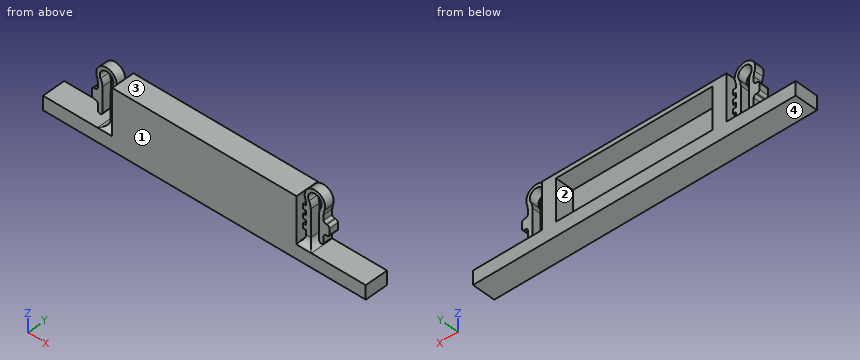
from build123d import *

# Parameters (mm, degrees)
BOSS_EXTRUDE1_DEPTH = 12.7
SKETCH6_W           = 86.36
SKETCH6_H           = 22.86
CUT_EXTRUDE3_DEPTH  = 10.16
SKETCH7_W           = 12.7
SKETCH7_H           = 25.4
CUT_EXTRUDE4_DEPTH  = 12.7
SKETCH14_W          = 88.9
SKETCH14_H          = 33.02
CUT_EXTRUDE5_DEPTH  = 19.558
BOSS_EXTRUDE2_START = -3.81
SKETCH15_W          = 2.54
SKETCH15_H          = 21.363451449
SKETCH15_W_2        = 3.175
SKETCH15_H_2        = 5.842
BOSS_EXTRUDE2_DEPTH = 5.08
FILLET1_R           = 7.62
FILLET2_R           = 1.27
FILLET3_R           = 3.81
BOSS_EXTRUDE3_START = -3.81
SKETCH16_W          = 1.778
SKETCH16_H          = 2.54
BOSS_EXTRUDE3_DEPTH = 5.08


# Some blends are built 0.0001 mm under size
with BuildPart() as part:
    # Sketch1 → Boss-Extrude1 (new body)
    with BuildSketch(Plane(origin=(0, 0, 0), x_dir=(1, 0, 0), z_dir=(0, 1, 0))):
        Polygon((88.9, 16.51), (-88.9, 16.51), (-88.9, 8.89), (-63.5, 8.89), (-63.5, -16.51), (63.5, -16.51), (63.5, 8.89), (88.9, 8.89), align=None)
    extrude(amount=BOSS_EXTRUDE1_DEPTH)

    # Sketch6 → Cut-Extrude3 (cut)
    with BuildSketch(Plane(origin=(0, 12.7, 0), x_dir=(1, 0, 0), z_dir=(0, 1, 0))):
        with Locations((0, -2.54)):
            Rectangle(SKETCH6_W, SKETCH6_H)
    extrude(amount=-CUT_EXTRUDE3_DEPTH, mode=Mode.SUBTRACT)

    # Sketch7 → Cut-Extrude4 (cut)
    with BuildSketch(Plane(origin=(0, 12.7, 0), x_dir=(1, 0, 0), z_dir=(0, 1, 0))):
        with Locations((57.15, -3.81)):
            Rectangle(SKETCH7_W, SKETCH7_H)
        with Locations((-57.15, -3.81)):
            Rectangle(SKETCH7_W, SKETCH7_H)
    extrude(amount=-CUT_EXTRUDE4_DEPTH, mode=Mode.SUBTRACT)

    # Sketch14 → Cut-Extrude5 (cut)
    with BuildSketch(Plane(origin=(0, 12.7, 0), x_dir=(1, 0, 0), z_dir=(0, 1, 0))):
        with Locations((44.45, 0)):
            Rectangle(SKETCH14_W, SKETCH14_H)
    extrude(amount=-CUT_EXTRUDE5_DEPTH, mode=Mode.SUBTRACT)

    # Sketch15 → Boss-Extrude2 (add)
    with BuildSketch(Plane(origin=(0, 12.7, 0), x_dir=(1, 0, 0), z_dir=(0, 1, 0)).offset(BOSS_EXTRUDE2_START)):
        with Locations((-53.848, -1.791725725)):
            Rectangle(SKETCH15_W, SKETCH15_H)
        with BuildLine():
            ThreePointArc((-59.69, -12.473451449), (-57.404, -19.184020308), (-55.118, -12.473451449))
            Line((-55.118, -12.473451449), (-52.578, -12.473451449))
            ThreePointArc((-52.578, -12.473451449), (-57.404, -21.103897158), (-62.23, -12.473451449))
            Line((-62.23, -12.473451449), (-62.23, 5.125982646))
            Line((-62.23, 5.125982646), (-59.69, 5.125982646))
            Line((-59.69, 5.125982646), (-59.69, -12.473451449))
        make_face()
        with Locations((-63.8175, -3.758774926)):
            Rectangle(SKETCH15_W_2, SKETCH15_H_2)
    extrude(amount=-BOSS_EXTRUDE2_DEPTH)

    # Fillet1
    fillet1_edges = [part.edges().sort_by_distance(p)[0] for p in [
        (-59.69, 6.35, 12.473451449),
        (-55.118, 6.35, 12.473451449),
        (-62.23, 6.35, 12.473451449),
        (-52.578, 6.35, 12.473451449),
    ]]
    fillet(fillet1_edges, radius=FILLET1_R)

    # Fillet2
    fillet2_edges = [part.edges().sort_by_distance(p)[0] for p in [
        (-62.23, 6.35, 6.679774926),
        (-65.405, 6.35, 6.679774926),
        (-65.405, 6.35, 0.837774926),
        (-62.23, 6.35, 0.837774926),
        (-59.69, 6.35, -5.125982646),
        (-62.23, 6.35, -5.125982646),
    ]]
    fillet(fillet2_edges, radius=FILLET2_R - 0.0001)  # a hair under: the kernel refuses the full size

    # Fillet3
    # the kernel refuses this fillet: 3.81 mm, written as the material it adds along each edge
    with BuildSketch(Plane(origin=(-52.578, 8.89, -8.89), x_dir=(0, 0, 1), z_dir=(0, -1, 0)), Plane(origin=(-55.118, 8.89, -8.89), x_dir=(-1, 0, 0), z_dir=(0, -1, 0))) as fillet3_piece_1:
        with BuildLine():
            CenterArc((FILLET3_R, -FILLET3_R), FILLET3_R, 90, 90)
            Line((0, -FILLET3_R), (-FILLET3_R * 0.02, -FILLET3_R))
            Line((-FILLET3_R * 0.02, -FILLET3_R), (-FILLET3_R * 0.02, FILLET3_R * 0.02))
            Line((-FILLET3_R * 0.02, FILLET3_R * 0.02), (FILLET3_R, FILLET3_R * 0.02))
            Line((FILLET3_R, FILLET3_R * 0.02), (FILLET3_R, 0))
        make_face()
    extrude(amount=5.08)
    with BuildSketch(Plane(origin=(-52.578, 3.81, -8.89), x_dir=(0, -1, 0), z_dir=(-1, 0, 0)), Plane(origin=(-52.578, 8.89, -8.89), x_dir=(0, 0, 1), z_dir=(-1, 0, 0))) as fillet3_piece_2:
        with BuildLine():
            CenterArc((FILLET3_R, FILLET3_R), FILLET3_R, 180, 90)
            Line((0, FILLET3_R), (-FILLET3_R * 0.02, FILLET3_R))
            Line((-FILLET3_R * 0.02, FILLET3_R), (-FILLET3_R * 0.02, -FILLET3_R * 0.02))
            Line((-FILLET3_R * 0.02, -FILLET3_R * 0.02), (FILLET3_R, -FILLET3_R * 0.02))
            Line((FILLET3_R, -FILLET3_R * 0.02), (FILLET3_R, 0))
        make_face()
    extrude(amount=2.54)
    with BuildSketch(Plane(origin=(-43.053, 8.89, -8.89), x_dir=(0, 0, 1), z_dir=(-1, 0, 0))) as fillet3_piece_3a_section:
        with BuildLine():
            CenterArc((FILLET3_R, FILLET3_R), FILLET3_R, 180, 90)
            Line((0, FILLET3_R), (-FILLET3_R * 0.02, FILLET3_R))
            Line((-FILLET3_R * 0.02, FILLET3_R), (-FILLET3_R * 0.02, -FILLET3_R * 0.02))
            Line((-FILLET3_R * 0.02, -FILLET3_R * 0.02), (FILLET3_R, -FILLET3_R * 0.02))
            Line((FILLET3_R, -FILLET3_R * 0.02), (FILLET3_R, 0))
        make_face()
    fillet3_piece_3a = extrude(amount=12.065, mode=Mode.PRIVATE)
    fillet3_piece_3a = split(fillet3_piece_3a, bisect_by=Plane(origin=(-52.578, 9.752565385, -8.027434615), z_dir=(1, 0, 0)), keep=Keep.TOP, mode=Mode.PRIVATE)
    with BuildSketch(Plane(origin=(-52.578, 18.415, -8.89), x_dir=(0, 0, 1), z_dir=(0, -1, 0))) as fillet3_piece_3b_section:
        with BuildLine():
            CenterArc((FILLET3_R, -FILLET3_R), FILLET3_R, 90, 90)
            Line((0, -FILLET3_R), (-FILLET3_R * 0.02, -FILLET3_R))
            Line((-FILLET3_R * 0.02, -FILLET3_R), (-FILLET3_R * 0.02, FILLET3_R * 0.02))
            Line((-FILLET3_R * 0.02, FILLET3_R * 0.02), (FILLET3_R, FILLET3_R * 0.02))
            Line((FILLET3_R, FILLET3_R * 0.02), (FILLET3_R, 0))
        make_face()
    fillet3_piece_3b = extrude(amount=14.605, mode=Mode.PRIVATE)
    fillet3_piece_3b = split(fillet3_piece_3b, bisect_by=Plane(origin=(-51.715434615, 8.89, -8.027434615), z_dir=(0, 1, 0)), keep=Keep.TOP, mode=Mode.PRIVATE)
    fillet3_piece_3 = fillet3_piece_3a & fillet3_piece_3b
    add(fillet3_piece_3)
    with BuildSketch(Plane(origin=(-52.578, 8.89, -8.89), x_dir=(0, 0, 1), z_dir=(0, -1, 0))) as fillet3_piece_4a_section:
        with BuildLine():
            CenterArc((FILLET3_R, -FILLET3_R), FILLET3_R, 90, 90)
            Line((0, -FILLET3_R), (-FILLET3_R * 0.02, -FILLET3_R))
            Line((-FILLET3_R * 0.02, -FILLET3_R), (-FILLET3_R * 0.02, FILLET3_R * 0.02))
            Line((-FILLET3_R * 0.02, FILLET3_R * 0.02), (FILLET3_R, FILLET3_R * 0.02))
            Line((FILLET3_R, FILLET3_R * 0.02), (FILLET3_R, 0))
        make_face()
    fillet3_piece_4a = extrude(amount=14.605, mode=Mode.PRIVATE)
    fillet3_piece_4a = split(fillet3_piece_4a, bisect_by=Plane(origin=(-51.715434615, 3.81, -8.027434615), z_dir=(0, -1, 0)), keep=Keep.TOP, mode=Mode.PRIVATE)
    with BuildSketch(Plane(origin=(-43.053, 3.81, -8.89), x_dir=(0, -1, 0), z_dir=(-1, 0, 0))) as fillet3_piece_4b_section:
        with BuildLine():
            CenterArc((FILLET3_R, FILLET3_R), FILLET3_R, 180, 90)
            Line((0, FILLET3_R), (-FILLET3_R * 0.02, FILLET3_R))
            Line((-FILLET3_R * 0.02, FILLET3_R), (-FILLET3_R * 0.02, -FILLET3_R * 0.02))
            Line((-FILLET3_R * 0.02, -FILLET3_R * 0.02), (FILLET3_R, -FILLET3_R * 0.02))
            Line((FILLET3_R, -FILLET3_R * 0.02), (FILLET3_R, 0))
        make_face()
    fillet3_piece_4b = extrude(amount=12.065, mode=Mode.PRIVATE)
    fillet3_piece_4b = split(fillet3_piece_4b, bisect_by=Plane(origin=(-52.578, 2.947434615, -8.027434615), z_dir=(1, 0, 0)), keep=Keep.TOP, mode=Mode.PRIVATE)
    fillet3_piece_4 = fillet3_piece_4a & fillet3_piece_4b
    add(fillet3_piece_4)
    with BuildSketch(Plane(origin=(-52.578, 8.89, -8.89), x_dir=(0, 0, 1), z_dir=(-1, 0, 0))) as fillet3_piece_5a_section:
        with BuildLine():
            CenterArc((FILLET3_R, FILLET3_R), FILLET3_R, 180, 90)
            Line((0, FILLET3_R), (-FILLET3_R * 0.02, FILLET3_R))
            Line((-FILLET3_R * 0.02, FILLET3_R), (-FILLET3_R * 0.02, -FILLET3_R * 0.02))
            Line((-FILLET3_R * 0.02, -FILLET3_R * 0.02), (FILLET3_R, -FILLET3_R * 0.02))
            Line((FILLET3_R, -FILLET3_R * 0.02), (FILLET3_R, 0))
        make_face()
    fillet3_piece_5a = extrude(amount=12.065, mode=Mode.PRIVATE)
    fillet3_piece_5a = split(fillet3_piece_5a, bisect_by=Plane(origin=(-55.118, 9.752565385, -8.027434615), z_dir=(-1, 0, 0)), keep=Keep.TOP, mode=Mode.PRIVATE)
    with BuildSketch(Plane(origin=(-55.118, 18.415, -8.89), x_dir=(-1, 0, 0), z_dir=(0, -1, 0))) as fillet3_piece_5b_section:
        with BuildLine():
            CenterArc((FILLET3_R, -FILLET3_R), FILLET3_R, 90, 90)
            Line((0, -FILLET3_R), (-FILLET3_R * 0.02, -FILLET3_R))
            Line((-FILLET3_R * 0.02, -FILLET3_R), (-FILLET3_R * 0.02, FILLET3_R * 0.02))
            Line((-FILLET3_R * 0.02, FILLET3_R * 0.02), (FILLET3_R, FILLET3_R * 0.02))
            Line((FILLET3_R, FILLET3_R * 0.02), (FILLET3_R, 0))
        make_face()
    fillet3_piece_5b = extrude(amount=14.605, mode=Mode.PRIVATE)
    fillet3_piece_5b = split(fillet3_piece_5b, bisect_by=Plane(origin=(-55.980565385, 8.89, -8.027434615), z_dir=(0, 1, 0)), keep=Keep.TOP, mode=Mode.PRIVATE)
    fillet3_piece_5 = fillet3_piece_5a & fillet3_piece_5b
    add(fillet3_piece_5)
    with BuildSketch(Plane(origin=(-52.578, 3.81, -8.89), x_dir=(0, -1, 0), z_dir=(-1, 0, 0))) as fillet3_piece_6a_section:
        with BuildLine():
            CenterArc((FILLET3_R, FILLET3_R), FILLET3_R, 180, 90)
            Line((0, FILLET3_R), (-FILLET3_R * 0.02, FILLET3_R))
            Line((-FILLET3_R * 0.02, FILLET3_R), (-FILLET3_R * 0.02, -FILLET3_R * 0.02))
            Line((-FILLET3_R * 0.02, -FILLET3_R * 0.02), (FILLET3_R, -FILLET3_R * 0.02))
            Line((FILLET3_R, -FILLET3_R * 0.02), (FILLET3_R, 0))
        make_face()
    fillet3_piece_6a = extrude(amount=12.065, mode=Mode.PRIVATE)
    fillet3_piece_6a = split(fillet3_piece_6a, bisect_by=Plane(origin=(-55.118, 2.947434615, -8.027434615), z_dir=(-1, 0, 0)), keep=Keep.TOP, mode=Mode.PRIVATE)
    with BuildSketch(Plane(origin=(-55.118, 8.89, -8.89), x_dir=(-1, 0, 0), z_dir=(0, -1, 0))) as fillet3_piece_6b_section:
        with BuildLine():
            CenterArc((FILLET3_R, -FILLET3_R), FILLET3_R, 90, 90)
            Line((0, -FILLET3_R), (-FILLET3_R * 0.02, -FILLET3_R))
            Line((-FILLET3_R * 0.02, -FILLET3_R), (-FILLET3_R * 0.02, FILLET3_R * 0.02))
            Line((-FILLET3_R * 0.02, FILLET3_R * 0.02), (FILLET3_R, FILLET3_R * 0.02))
            Line((FILLET3_R, FILLET3_R * 0.02), (FILLET3_R, 0))
        make_face()
    fillet3_piece_6b = extrude(amount=14.605, mode=Mode.PRIVATE)
    fillet3_piece_6b = split(fillet3_piece_6b, bisect_by=Plane(origin=(-55.980565385, 3.81, -8.027434615), z_dir=(0, -1, 0)), keep=Keep.TOP, mode=Mode.PRIVATE)
    fillet3_piece_6 = fillet3_piece_6a & fillet3_piece_6b
    add(fillet3_piece_6)

    # Sketch16 → Boss-Extrude3 (add)
    with BuildSketch(Plane(origin=(0, 12.7, 0), x_dir=(1, 0, 0), z_dir=(0, 1, 0)).offset(BOSS_EXTRUDE3_START)):
        with Locations((-51.689, 1.27)):
            Rectangle(SKETCH16_W, SKETCH16_H)
        with Locations((-51.689, -3.81)):
            Rectangle(SKETCH16_W, SKETCH16_H)
        with Locations((-51.689, -8.89)):
            Rectangle(SKETCH16_W, SKETCH16_H)
    extrude(amount=-BOSS_EXTRUDE3_DEPTH)

    # Mirror1: part across plane


with BuildPart() as part_1:
    add(part.part)
    add(part.part.mirror(Plane(origin=(0, -6.858, -16.51), x_dir=(0, 0, 1), z_dir=(-1, 0, 0))))


solid = part_1.part
Part model, mm, in its own coordinate system. Face numbers are marked on the shaded views. A direction names the side the tool comes from. Coordinates: 2 decimals unless noted, no trailing zeros. Loops run counter-clockwise (first coordinate to the right, second up) from the corner with the lowest first, then second, coordinate; pieces in that order, holes last. Notation, with made-up numbers: (52, 36.5) -> (106, 36.5) arc R9 ccw to (106, 42.5) -> close; hole circle Ø9 at (53.5, 55). An arc over 180 degrees is marked (long way). Use a Markdown table: item, result. Add a question column.
Item 1: Probe probe 1 along Z at (x, y) = (2.5, 7.25); probe 2 along X at (y, z) = (5.75, 6.5); probe 3 along Y at (x, z) = (-18, 5). List the from-to ranges inside material, lowest first.
Item 2: Pull direction X, two halves, no side cores. Call the marked faces 3 and 4: +X half, -X half, draft (parallel to the pull), parting line (faces both ways), or undercut.
Item 3: Flat gauge pins, fed straight in: P1, Ø4, axis at y = 9.5, z = 13.5, coming from the +X side; P2, Ø0.5, axis at x = -52, y = 5, coming from the +Z side; P3, Ø3, axis at y = 9.5, z = -5, coming from the -X side; P4, Ø5, axis at x = 68.5, z = -5.5, coming from the -Y side. Where does each tip first touch, or does it go through?
Item 4: Band-saw the part on B-B on y = 5.5. Give the number of separate pieces and of enclosed holes in the cut face, plus the area to 3 significant figures.
Item 5: Band-saw the part on A-A on x = 6. Write the cut outline in (y, z), plus the area to 3 significant figures.
Item 6: Which spindle directions (+Z, -Z, +X, -X, +Y, -Y) get a long thin tool onto all of the face, cutting with end or side? Do the marked faces 1 and 2. Say none if no direction does.
Geometry says:
| question | item | result |
|---|---|---|
| 1 | probe 1 | -16.51 to -8.89, 13.97 to 16.51 |
| 1 | probe 2 | -64.79 to -59.69, -55.12 to -52.58, -50.8 to -43.18, 43.18 to 50.8, 52.58 to 55.12, 59.69 to 64.79 |
| 1 | probe 3 | 0 to 2.54 |
| 2 | face 3 | undercut |
| 2 | face 4 | draft |
| 3 | P1 | x = 63.07 |
| 3 | P2 | z = 17.79 |
| 3 | P3 | x = -62.23 |
| 3 | P4 | through |
| 4 | separate pieces | 1 |
| 4 | enclosed holes | 7 |
| 4 | area | 2,310 mm² |
| 5 | outline | (0, -16.51) -> (12.7, -16.51) -> (12.7, -8.89) -> (2.54, -8.89) -> (2.54, 13.97) -> (12.7, 13.97) -> (12.7, 16.51) -> (0, 16.51) -> close |
| 5 | area | 187 mm² |
| 6 | face 1 | +Z, -Z, +X, -X, -Y |
| 6 | face 2 | +Y |
